Source: CAD feature listing. Evaluate the final solid. Frame: model axes, mm. A direction names the side the tool comes from. Round coordinates to 2 decimals unless told otherwise and drop trailing zeros. Loops run counter-clockwise (first coordinate to the right, second up) from the corner with the lowest first, then second, coordinate; pieces in that order, holes last.
Item 1: Section query C-C on z = 2.5. Return loops of the section in (x, y), then the cut area to 3 significant figures.
Item 2: Access query for faces 1 (the flat face through (1, -113.652, 4)), 2 (the flat face through (1, 2, 0.152)). Directions: +Z, -Z, +X, -X, +Y, -Y. A direction counts if a zero-diameter tool reaches every point of the face in a straight line with its end or side. Return the directions, or none.
Item 3: Ray query, L1, parallel to Y at x = -83.72, z = 0.1; L2, parallel to X at y = -59, z = 6.25; L3, parallel to Y at x = -17, z = 5.5. Return the intervals inside material, ascending.
Item 4: First-contact query: P1, Ø1.5, axis at x = 16, y = -13, coming from the +Z side; P2, Ø2, axis at x = -29.5, z = 4, coming from the +Y side. Flat tips, straight axial feed; report the tip coordinate or a pass-through.
Item 5: Section query A-A on y = -1.5. Return loops of the section in (x, z), then the cut area to 3 significant figures.
Item 6: Section query B-B on x = 16.5. Return loops of the section in (y, z).
```python
from build123d import *

# Parameters (mm, degrees)
SKETCH1_W            = 89.72
SKETCH1_H            = 227
SKETCH1_R            = 2
HEAT_EXCHANGER_DEPTH = 0.1524
CONVECTION_FIN_DEPTH = 7.2048


with BuildPart() as part:
    # Sketch1 → Heat Exchanger (new body)
    with BuildSketch(Plane.XY):
        with Locations((-44.86, 0)):
            Rectangle(SKETCH1_W, SKETCH1_H)
        with Locations((-83.72, -56.6738)):
            Circle(SKETCH1_R, mode=Mode.SUBTRACT)
        with Locations((-83.72, 56.9786)):
            Circle(SKETCH1_R, mode=Mode.SUBTRACT)
    heat_exchanger = extrude(amount=HEAT_EXCHANGER_DEPTH)

    # Sketch3 → Convection Fin (add)
    with BuildSketch(Plane.XY):
        Polygon((0, -113.6524), (0, -113.5), (-89.72, -113.5), (-89.72, 113.5), (-89.8724, 113.5), (-89.8724, -113.6524), align=None)
    convection_fin = extrude(amount=CONVECTION_FIN_DEPTH)

    # Mirror1: Heat Exchanger, Convection Fin across plane
    add(heat_exchanger.mirror(Plane(origin=(0, 0, 0), x_dir=(0, 0, 1), z_dir=(1, 0, 0))))
    add(convection_fin.mirror(Plane(origin=(0, 0, 0), x_dir=(0, 0, 1), z_dir=(1, 0, 0))))


solid = part.part
```
Data:
1. outline: (-89.87, -113.65) - (89.87, -113.65) - (89.87, 113.5) - (89.72, 113.5) - (89.72, -113.5) - (-89.72, -113.5) - (-89.72, 113.5) - (-89.87, 113.5) - close
1. area: 96.6 mm2
2. face 1: +Z, -Z, +X, -X, -Y
2. face 2: +Z, +Y
3. L1: y = -113.65 to -58.67, -54.67 to 54.98, 58.98 to 113.5
3. L2: x = -89.87 to -89.72, 89.72 to 89.87
3. L3: y = -113.65 to -113.5
4. P1: stops at z = 0.15
4. P2: stops at y = -113.5
5. outline: (-89.87, 0) - (89.87, 0) - (89.87, 7.2) - (89.72, 7.2) - (89.72, 0.15) - (-89.72, 0.15) - (-89.72, 7.2) - (-89.87, 7.2) - close
5. area: 29.5 mm2
6. outline: (-113.65, 0) - (113.5, 0) - (113.5, 0.15) - (-113.5, 0.15) - (-113.5, 7.2) - (-113.65, 7.2) - close
